Geometry check sheet. Reference: the model listing, model coordinates, mm. A direction names the side the tool comes from. Round coordinates to 2 decimals unless told otherwise and drop trailing zeros. Order: outer loops, then holes, each group sorted by start corner. A loop starts at its lowest first (then second) coordinate and runs counter-clockwise, first axis right, second up.
(1) Cross-section at B-B on x = -37. Enter the section's corners in (y, z).
(2) Cross-section at D-D on x = -45. Enter the section's corners in (y, z).
(3) Thickness scan on L1, parallel to X at y = -14.5, z = 5; L2, parallel to Y at x = -61.65, z = 19.05; L3, parallel to Z at x = -61, y = -17. Record the ranges inside material, lowest first.
(4) Gauge pin test, flat ends, axial feed: P1, Ø3, axis at y = -16.85, z = 50.8, coming from the -X side; P2, Ø5.5, axis at x = -52.39, z = 5.72, coming from the -Y side; P3, Ø1.6, axis at y = -30.32, z = 52.19, coming from the +X side. Record the tip position at first contact, or that the pin passes through.
(5) Set-up check for faces 1 (the face through (-56.247, -7.56, 56.244)), 2 (the face through (-62.392, -15.687, 20.323)), 3 (the face through (-54.034, -9.835, 6.234)), 4 (the face through (-64.452, -20, 34)): record each of +Z, -Z, +X, -X, +Y, -Y from which the full face is reachable in a straight line by a thin tool's end or side.
(6) Cross-section at A-A on y = -27.25. Enter the section's corners in (x, z), and give its area (3 significant figures).
(7) Cross-section at C-C on z = 61.5. Enter the section's corners in (x, y).
(8) Draft check along Z on faces 5 (the face through (-13.652, -24, 34)), 6 (the face through (-36, -11, 69.85)), 7 (the face through (-57.65, -9.855, 56.632)). Enter one of: pulls with the +Z half, pulls with the -Z half, needs draft (parallel to the pull), parting line crosses it, or undercut.
from build123d import *

# Parameters (mm, degrees)
BOSS_EXTRUDE1_DEPTH             = 69.85
TAP_DRILL_FOR_1_2_20_TAP1_D     = 11.50874
TAP_DRILL_FOR_1_2_20_TAP1_DEPTH = 12.7
TAP_DRILL_FOR_1_2_20_TAP1_TIP   = 3.45757432
LPATTERN2_COUNT                 = 2
LPATTERN2_PITCH                 = 43.18
LPATTERN2_COUNT_DIR2            = 2
LPATTERN2_PITCH_DIR2            = 43.18
TAP_DRILL_FOR_8_32_TAP1_D       = 3.4544
TAP_DRILL_FOR_8_32_TAP1_DEPTH   = 4.826
TAP_DRILL_FOR_8_32_TAP1_TIP     = 1.037806461
TAP_DRILL_FOR_8_32_TAP4_D       = 3.4544
TAP_DRILL_FOR_8_32_TAP4_DEPTH   = 4.064
TAP_DRILL_FOR_8_32_TAP4_TIP     = 1.037806461
TAP_DRILL_FOR_6_32_TAP1_D       = 2.7051
TAP_DRILL_FOR_6_32_TAP1_DEPTH   = 5.08
TAP_DRILL_FOR_6_32_TAP1_TIP     = 0.81269403


with BuildPart() as part:
    # Sketch1 → Boss-Extrude1 (new body)
    with BuildSketch(Plane.XY):
        with BuildLine():
            Line((-64.452009828, -5.932047122), (-64.452009828, -35.142047122))
            Line((-64.452009828, -35.142047122), (-58.102009828, -35.142047122))
            Line((-58.102009828, -35.142047122), (-58.102009828, -13.552047122))
            ThreePointArc((-58.102009828, -13.552047122), (-57.73003544, -12.65402151), (-56.832009828, -12.282047122))
            Line((-56.832009828, -12.282047122), (-14.922009828, -12.282047122))
            ThreePointArc((-14.922009828, -12.282047122), (-14.023984216, -12.65402151), (-13.652009828, -13.552047122))
            Line((-13.652009828, -13.552047122), (-13.652009828, -35.142047122))
            Line((-13.652009828, -35.142047122), (-7.302009828, -35.142047122))
            Line((-7.302009828, -35.142047122), (-7.302009828, -5.932047122))
            Line((-7.302009828, -5.932047122), (-64.452009828, -5.932047122))
        make_face()
    extrude(amount=BOSS_EXTRUDE1_DEPTH)

    # Tap Drill for 1/2-20 Tap1
    with Locations(Plane(origin=(0, -5.932047122, 0), x_dir=(-1, 0, 0), z_dir=(0, 1, 0))):
        with Locations((35.877009828, 34.925)):
            Hole(TAP_DRILL_FOR_1_2_20_TAP1_D / 2, depth=TAP_DRILL_FOR_1_2_20_TAP1_DEPTH)
            with Locations((0, 0, -(TAP_DRILL_FOR_1_2_20_TAP1_DEPTH + TAP_DRILL_FOR_1_2_20_TAP1_TIP / 2))):  # 118° drill point
                Cone(0, TAP_DRILL_FOR_1_2_20_TAP1_D / 2, TAP_DRILL_FOR_1_2_20_TAP1_TIP, mode=Mode.SUBTRACT)

    # Sketch10 → Tap Drill for M3x0.5 Tap1 (revolve, cut)
    with BuildSketch(Plane(origin=(-57.467009828, -5.932047122, 13.335), x_dir=(0, 0, 1), z_dir=(1, 0, 0))):
        Polygon((0, 0), (0, 4.053075774), (1.25, 3.302), (1.25, 0), align=None)
    tap_drill_for_m3x0_5_tap1 = revolve(axis=Axis((-57.467009828, 0.417952878, 13.335), (0, -1, 0)), mode=Mode.SUBTRACT)

    # LPattern2: Tap Drill for M3x0.5 Tap1 2 × 2
    with Locations(*[(i * LPATTERN2_PITCH, 0, j * LPATTERN2_PITCH_DIR2) for i in range(LPATTERN2_COUNT) for j in range(LPATTERN2_COUNT_DIR2) if (i, j) != (0, 0)]):
        add(tap_drill_for_m3x0_5_tap1, mode=Mode.SUBTRACT)

    # Tap Drill for #8-32 Tap1
    with Locations(Plane.XZ.offset(12.282047122)):
        with Locations((-52.387009828, 64.135), (-19.367009828, 64.135), (-52.387009828, 5.715), (-19.367009828, 5.715)):
            Hole(TAP_DRILL_FOR_8_32_TAP1_D / 2, depth=TAP_DRILL_FOR_8_32_TAP1_DEPTH)
            with Locations((0, 0, -(TAP_DRILL_FOR_8_32_TAP1_DEPTH + TAP_DRILL_FOR_8_32_TAP1_TIP / 2))):  # 118° drill point
                Cone(0, TAP_DRILL_FOR_8_32_TAP1_D / 2, TAP_DRILL_FOR_8_32_TAP1_TIP, mode=Mode.SUBTRACT)

    # Tap Drill for #8-32 Tap4
    with Locations(Plane.ZY.offset(64.452009828)):
        with Locations((19.05, -16.854047122), (50.8, -16.854047122)):
            Hole(TAP_DRILL_FOR_8_32_TAP4_D / 2, depth=TAP_DRILL_FOR_8_32_TAP4_DEPTH)
            with Locations((0, 0, -(TAP_DRILL_FOR_8_32_TAP4_DEPTH + TAP_DRILL_FOR_8_32_TAP4_TIP / 2))):  # 118° drill point
                Cone(0, TAP_DRILL_FOR_8_32_TAP4_D / 2, TAP_DRILL_FOR_8_32_TAP4_TIP, mode=Mode.SUBTRACT)

    # Tap Drill for #6-32 Tap1
    with Locations(Plane(origin=(-7.302009828, 0, 0), x_dir=(0, 0, -1), z_dir=(1, 0, 0))):
        with Locations((-52.1890625, -30.316047122), (-17.6609375, -30.316047122)):
            Hole(TAP_DRILL_FOR_6_32_TAP1_D / 2, depth=TAP_DRILL_FOR_6_32_TAP1_DEPTH)
            with Locations((0, 0, -(TAP_DRILL_FOR_6_32_TAP1_DEPTH + TAP_DRILL_FOR_6_32_TAP1_TIP / 2))):  # 118° drill point
                Cone(0, TAP_DRILL_FOR_6_32_TAP1_D / 2, TAP_DRILL_FOR_6_32_TAP1_TIP, mode=Mode.SUBTRACT)


solid = part.part
Found:
1. outline: (-12.28, 0) - (-5.93, 0) - (-5.93, 29.28) - (-12.28, 29.28) - close; (-12.28, 40.57) - (-5.93, 40.57) - (-5.93, 69.85) - (-12.28, 69.85) - close
2. outline: (-12.28, 0) - (-5.93, 0) - (-5.93, 69.85) - (-12.28, 69.85) - close
3. L1: x = -64.45 to -58.1, -13.65 to -7.3
3. L2: y = -35.14 to -18.58, -15.13 to -5.93
3. L3: z = 0 to 17.33, 20.77 to 49.08, 52.52 to 69.85
4. P1: stops at x = -60.25
4. P2: stops at y = -12.28
4. P3: stops at x = -12.71
5. face 1: +Y
5. face 2: -X
5. face 3: -Y
5. face 4: +Z, -Z, -X, +Y, -Y
6. outline: (-64.45, 0) - (-58.1, 0) - (-58.1, 69.85) - (-64.45, 69.85) - close; (-13.65, 0) - (-7.3, 0) - (-7.3, 69.85) - (-13.65, 69.85) - close
6. area: 887 mm2
7. outline: (-64.45, -35.14) - (-58.1, -35.14) - (-58.1, -13.55) arc R1.27 cw to (-56.83, -12.28) - (-14.92, -12.28) arc R1.27 cw to (-13.65, -13.55) - (-13.65, -35.14) - (-7.3, -35.14) - (-7.3, -5.93) - (-64.45, -5.93) - close
8. face 5: needs draft
8. face 6: pulls with the +Z half
8. face 7: undercut
